Design review of the part built by this model. Coordinates are the model's own, in mm. A direction names the side the tool comes from. Coordinates: 2 decimals unless noted, no trailing zeros. Loops run counter-clockwise (first coordinate to the right, second up) from the corner with the lowest first, then second, coordinate; pieces in that order, holes last. Notation, with made-up numbers: (21.5, 43.5) -> (46.5, 43.5) arc R35 ccw to (46.5, 79.5) -> close; hole circle Ø4 at (-7, -13). An arc over 180 degrees is marked (long way). Use one line per item in the form item = value. Start each with the question number.
1. Consider section C-C (z = 2). State the section outline as (x, y) points.
2. Consider section B-B (y = 5.5). State the section outline as (x, z) points.
3. Consider section A-A (x = 0). State how many separate pieces and enclosed holes the cut face has, then the cut area to 3 significant figures.
4. The part is to be moulded in two halves that separate along Z. For faces 1 (the face through (2.38, 1.29, 1.17)), 2 (the face through (0, -5, -5.5)), 3 (the face through (3, 0, 5.5)), say which applies: released by +Z, released by -Z, zero draft, split by the parting line, or undercut.
5. Consider section D-D (z = -3.75). State the section outline as (x, y) points (3 decimals), then the cut area to 3 significant figures.
6. For pin 1 (1.6 mm diameter, centred on y = 0, z = 1, fed in from -X); pin 2 (3.5 mm diameter, centred on y = 0, z = 1, fed in from -X); pin 3 (1 mm diameter, centred on x = 6, z = -2.5, fed in from -Y); pin 4 (2 mm diameter, centred on x = 1.5, z = 0, fed in from +Y), all flat-tipped, find the tip position at first contact; note any pin that passes through.
7. Machinability: for faces 4 (the face through (2, -2, -2.65)), 5 (the face through (-2.71, 2.28, 4.51)), 6 (the face through (0, -5, -2.5)), which of the approach directions +Z, -Z, +X, -X, +Y, -Y give a long, thin tool a straight path to every point of the face, cutting with its end or side? Answer none if there is none.
8. Wall thickness on line 1 (Y direction, x = 0, z = -3.9) (3 decimals); line 2 (Y direction, x = 2.55, z = 1); line 3 (X direction, y = -1.5, z = 1): over which ranges is each line inside the solid? List them lowest first. Write a range as from..to.
from build123d import *

# Parameters (mm, degrees)
SKETCH1_R                = 11
SKETCH1_R_2              = 4.175
MAIN_BODY_DEPTH          = 5.5
SKETCH2_R                = 4.175
SKETCH2_R_2              = 2.2
MAIN_BOLT_SURFACE_DEPTH  = 8.15
SKETCH7_R                = 1.175
CUT_EXTRUDE4_DEPTH       = 12
SKETCH8_R                = 2.05
CUT_EXTRUDE5_DEPTH       = 2
CUT_EXTRUDE9_START       = -2.5
SKETCH11_R               = 11
SKETCH11_R_2             = 3
CUT_EXTRUDE9_DEPTH       = 6
CUT_EXTRUDE10_REACH      = 13
SKETCH10_R               = 11
SKETCH10_R_2             = 6
FILLET2_R                = 1
SKETCH12_R               = 1.3
CUT_EXTRUDE12_DEPTH      = 12
CUT_EXTRUDE12_DEPTH_BACK = 12
SKETCH13_R               = 1.35
CUT_EXTRUDE13_DEPTH      = 5.5


with BuildPart() as part:
    # Sketch1 → Main Body (new body, symmetric)
    with BuildSketch(Plane.XY):
        Circle(SKETCH1_R)
        Circle(SKETCH1_R_2, mode=Mode.SUBTRACT)
    extrude(amount=MAIN_BODY_DEPTH, both=True)

    # Sketch2 → Main Bolt Surface (add)
    with BuildSketch(Plane.XY.offset(5.5)):
        Circle(SKETCH2_R)
        Circle(SKETCH2_R_2, mode=Mode.SUBTRACT)
    extrude(amount=-MAIN_BOLT_SURFACE_DEPTH)

    # Sketch7 → Cut-Extrude4 (cut, through all)
    with BuildSketch(Plane.XY.offset(5.5)):
        with Locations((0, -8)):
            Circle(SKETCH7_R)
        with Locations((0, 8)):
            Circle(SKETCH7_R)
    extrude(amount=-CUT_EXTRUDE4_DEPTH, mode=Mode.SUBTRACT)

    # Sketch8 → Cut-Extrude5 (cut)
    with BuildSketch(Plane.XY.offset(5.5)):
        with Locations((0, 8)):
            Circle(SKETCH8_R)
        with Locations((0, -8)):
            Circle(SKETCH8_R)
    extrude(amount=-CUT_EXTRUDE5_DEPTH, mode=Mode.SUBTRACT)

    # Sketch11 → Cut-Extrude9 (cut)
    with BuildSketch(Plane.XY.offset(CUT_EXTRUDE9_START)):
        Circle(SKETCH11_R)
        Circle(SKETCH11_R_2, mode=Mode.SUBTRACT)
    extrude(amount=CUT_EXTRUDE9_DEPTH, mode=Mode.SUBTRACT)

    # Sketch10 → Cut-Extrude10 (cut, up to next)
    with BuildSketch(Plane.XY.offset(5.5), mode=Mode.PRIVATE) as cut_extrude10_sk1:
        Circle(SKETCH10_R)
        Circle(SKETCH10_R_2, mode=Mode.SUBTRACT)
    cut_extrude10_tool1 = extrude(cut_extrude10_sk1.sketch, amount=-CUT_EXTRUDE10_REACH, mode=Mode.PRIVATE) & part.part
    add(cut_extrude10_tool1.solids().sort_by_distance((-10.688873, 0, 5.5))[0], mode=Mode.SUBTRACT)

    # Fillet2
    fillet2_edges = [part.edges().sort_by_distance(p)[0] for p in [
        (-3, 0, -2.5),
    ]]
    fillet(fillet2_edges, radius=FILLET2_R)

    # Sketch12 → Cut-Extrude12 (cut, two sides)
    with BuildSketch(Plane(origin=(0, 0, 0), x_dir=(0, 0, -1), z_dir=(1, 0, 0))) as cut_extrude12_sk:
        with Locations((-1, 0)):
            Circle(SKETCH12_R)
    extrude(amount=CUT_EXTRUDE12_DEPTH, mode=Mode.SUBTRACT)
    extrude(cut_extrude12_sk.sketch, amount=-CUT_EXTRUDE12_DEPTH_BACK, mode=Mode.SUBTRACT)

    # Sketch13 → Cut-Extrude13 (cut)
    with BuildSketch(Plane.XY.offset(5.5)):
        with Locations((-3.999386509, 1.877034489)):
            Circle(SKETCH13_R)
    extrude(amount=-CUT_EXTRUDE13_DEPTH, mode=Mode.SUBTRACT)


solid = part.part
Geometry check:
q1.outline = (-2.88, -0.83) arc R3 ccw to (2.88, -0.83) -> (2.04, -0.83) arc R2.2 cw to (-2.04, -0.83) -> close; (-2.88, 0.83) -> (-2.04, 0.83) arc R2.2 cw to (2.04, 0.83) -> (2.88, 0.83) arc R3 ccw to start
q2.outline = (-9.53, -5.5) -> (9.53, -5.5) -> (9.53, -2.5) -> (-9.53, -2.5) -> close; (-2.4, 3.5) -> (2.4, 3.5) -> (2.4, 5.5) -> (-2.4, 5.5) -> close
q3.separate_pieces = 4
q3.enclosed_holes = 0
q3.area = 52.5 mm²
q4.face_1 = undercut
q4.face_2 = released by -Z
q4.face_3 = released by +Z
q5.outline = circle Ø22 at (0, 0); hole circle Ø8.35 at (0, 0); hole circle Ø2.35 at (0, -8); hole circle Ø2.35 at (0, 8)
q5.area = 317 mm²
q6.pin_1 = through
q6.pin_2 = -3
q6.pin_3 = -9.53
q6.pin_4 = 2.96
q7.face_4 = -Z
q7.face_5 = +Z
q7.face_6 = none
q8.line_1 = -11..-9.175, -6.825..-4.175, 4.175..6.825, 9.175..11
q8.line_2 = -1.58..-1.3, 1.3..1.58
q8.line_3 = -2.6..-1.61, 1.61..2.6
